```python
from build123d import *

# Parameters (mm, degrees)
SKETCH1_R               = 6
BOSS_EXTRUDE1_DEPTH     = 12
CUT_EXTRUDE1_DEPTH      = 15.696938457
CUT_EXTRUDE1_DEPTH_BACK = 15.696938457
SKETCH2_W               = 7.5
SKETCH2_H               = 8.5
CUT_EXTRUDE2_DEPTH      = 15.696938457
CUT_EXTRUDE2_DEPTH_BACK = 15.696938457
SKETCH3_R               = 0.75
BOSS_EXTRUDE2_DEPTH     = 40


with BuildPart() as part:
    # Sketch1 → Boss-Extrude1 (new body)
    with BuildSketch(Plane(origin=(0, 0, 0), x_dir=(1, 0, 0), z_dir=(0, 1, 0))):
        with Locations(Location((0, 0, 0), (0, 0, 270))):
            Circle(SKETCH1_R)
    extrude(amount=BOSS_EXTRUDE1_DEPTH)

    # Sketch2 → Cut-Extrude1 (cut, two sides: drawn at the far end of the back side and taken through both)
    with BuildSketch(Plane(origin=(0, 0, 0), x_dir=(0, 0, -1), z_dir=(1, 0, 0)).offset(-CUT_EXTRUDE1_DEPTH_BACK)):
        with Locations((0, 7.75)):
            Rectangle(SKETCH2_W, SKETCH2_H)
    extrude(amount=CUT_EXTRUDE1_DEPTH + CUT_EXTRUDE1_DEPTH_BACK, mode=Mode.SUBTRACT)

    # Sketch3 → Cut-Extrude2 (cut, two sides: drawn at the far end of the back side and taken through both)
    with BuildSketch(Plane.XY.offset(-CUT_EXTRUDE2_DEPTH_BACK)):
        with BuildLine():
            Line((-3.15, 5), (-3.15, 8.85))
            ThreePointArc((-3.15, 8.85), (-2.227386361, 11.077386361), (0, 12))
            Line((0, 12), (-4.683748499, 12))
            Line((-4.683748499, 12), (-4.683748499, 3.5))
            Line((-4.683748499, 3.5), (-4.65, 3.5))
            ThreePointArc((-4.65, 3.5), (-3.589339828, 3.939339828), (-3.15, 5))
        make_face()
        with BuildLine():
            Line((4.683748499, 12), (0, 12))
            ThreePointArc((0, 12), (2.227386361, 11.077386361), (3.15, 8.85))
            Line((3.15, 8.85), (3.15, 5))
            ThreePointArc((3.15, 5), (3.589339828, 3.939339828), (4.65, 3.5))
            Line((4.65, 3.5), (4.683748499, 3.5))
            Line((4.683748499, 3.5), (4.683748499, 12))
        make_face()
        with Locations((0, 8.85)):
            Circle(SKETCH3_R)
    extrude(amount=CUT_EXTRUDE2_DEPTH + CUT_EXTRUDE2_DEPTH_BACK, mode=Mode.SUBTRACT)

    # Sketch4 → Boss-Extrude2 (add)
    with BuildSketch(Plane.XZ):
        with BuildLine():
            Line((-0.6, 3.5), (-0.6, 4.207433897))
            ThreePointArc((-0.6, 4.207433897), (-2.799894973, 3.19735643), (-4.091454509, 1.15))
            Line((-4.091454509, 1.15), (-3.5, 1.15))
            Line((-3.5, 1.15), (-3.5, -1.15))
            Line((-3.5, -1.15), (-4.091454509, -1.15))
            ThreePointArc((-4.091454509, -1.15), (-2.799894973, -3.19735643), (-0.6, -4.207433897))
            Line((-0.6, -4.207433897), (-0.6, -3.5))
            Line((-0.6, -3.5), (0.6, -3.5))
            Line((0.6, -3.5), (0.6, -4.207433897))
            ThreePointArc((0.6, -4.207433897), (2.799894973, -3.19735643), (4.091454509, -1.15))
            Line((4.091454509, -1.15), (3.5, -1.15))
            Line((3.5, -1.15), (3.5, 1.15))
            Line((3.5, 1.15), (4.091454509, 1.15))
            ThreePointArc((4.091454509, 1.15), (2.799894973, 3.19735643), (0.6, 4.207433897))
            Line((0.6, 4.207433897), (0.6, 3.5))
            Line((0.6, 3.5), (-0.6, 3.5))
        make_face()
    extrude(amount=BOSS_EXTRUDE2_DEPTH)


solid = part.part
```
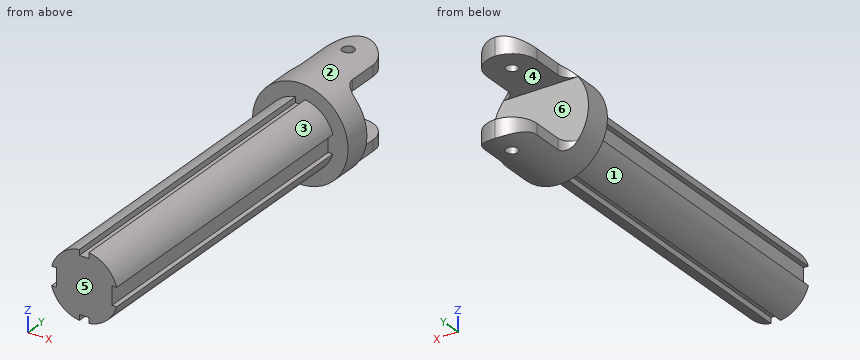
Check sheet for the modelled part. Datum: model origin and axes. Units: mm. Face numbers are marked on the shaded views. A direction names the side the tool comes from. Round coordinates to 2 decimals unless told otherwise and drop trailing zeros. Order: outer loops, then holes, each group sorted by start corner. A loop starts at its lowest first (then second) coordinate and runs counter-clockwise, first axis right, second up.
1) Tool access check on the marked faces 5 and 6. Record the directions out of +Z, -Z, +X, -X, +Y, -Y that give a thin tool (end or side, any length) a straight path to the whole face; none if there is none.
2) Go/stop test with flat-tipped pins: pin 1 Ø2 at (x, y) = (3.5, -13) entering from +Z; pin 2 Ø0.7 at (y, z) = (7.5, -4.5) entering from +X; pin 3 Ø1 at (x, y) = (0, -11) entering from -Z; pin 4 Ø1.4 at (x, y) = (0, 8.85) entering from -Z. Record where each tip stops, or that it passes through.
3) Section check A-A (y = -29.5). Record the boundary of the cut face in (x, z), and give its area (3 significant figures).
4) Section check D-D (x = -2.5). Record the boundary of the cut face in (y, z).
5) Mould release check, pull along Z, two halves, no side actions. Record for the marked faces 1, 2, 3 and 4: +Z half, -Z half, draft (parallel to the pull), parting line (faces both ways), or undercut.
6) Scan lines: line 1 (X direction, y = 8.85, z = -4.25); line 2 (Y direction, x = 0, z = -5); line 3 (Y direction, x = 1.5, z = -1.5). Record each from-to range of solid material in increasing order.
7) Section check B-B (z = 0). Record the boundary of the cut face in (x, y).
8) Section check C-C (x = 2.25). Record the boundary of the cut face in (y, z).
Result:
1. face 5: +Z, -Z, +X, -X, -Y
1. face 6: +X, -X, +Y
2. pin 1: stops at z = 3.44
2. pin 2: stops at x = 3.15
2. pin 3: stops at z = -3.5
2. pin 4: passes through
3. outline: (-4.09, -1.15) arc R4.25 ccw to (-0.6, -4.21) - (-0.6, -3.5) - (0.6, -3.5) - (0.6, -4.21) arc R4.25 ccw to (4.09, -1.15) - (3.5, -1.15) - (3.5, 1.15) - (4.09, 1.15) arc R4.25 ccw to (0.6, 4.21) - (0.6, 3.5) - (-0.6, 3.5) - (-0.6, 4.21) arc R4.25 ccw to (-4.09, 1.15) - (-3.5, 1.15) - (-3.5, -1.15) - close
3. area: 51.8 mm2
4. outline: (-40, -3.44) - (0, -3.44) - (0, -5.45) - (10.77, -5.45) - (10.77, -3.75) - (3.5, -3.75) - (3.5, 3.75) - (10.77, 3.75) - (10.77, 5.45) - (0, 5.45) - (0, 3.44) - (-40, 3.44) - close
5. face 1: -Z half
5. face 2: parting line
5. face 3: +Z half
5. face 4: undercut
6. line 1: x = -3.15 to -0.75, 0.75 to 3.15
6. line 2: y = 0 to 8.1, 9.6 to 12
6. line 3: y = -40 to 3.5
7. outline: (-6, 0) - (-3.5, 0) - (-3.5, -40) - (3.5, -40) - (3.5, 0) - (6, 0) - (6, 3.5) - (-6, 3.5) - close
8. outline: (-40, -3.61) - (0, -3.61) - (0, -5.56) - (11.05, -5.56) - (11.05, -3.75) - (3.5, -3.75) - (3.5, 3.75) - (11.05, 3.75) - (11.05, 5.56) - (0, 5.56) - (0, 3.61) - (-40, 3.61) - close
